Geometry check sheet. Reference: the model listing, model coordinates, mm. A direction names the side the tool comes from. Round coordinates to 2 decimals unless told otherwise and drop trailing zeros. Loops run counter-clockwise (first coordinate to the right, second up) from the corner with the lowest first, then second, coordinate; pieces in that order, holes last.
Autodesk Inventor part; units mm, degrees
ref_plane "YZ Plane" through (0, 0, 0) normal (1, 0, 0) x (0, 1, 0)
ref_plane "XZ Plane" through (0, 0, 0) normal (0, 1, 0) x (-1, 0, 0)
ref_plane "XY Plane" through (0, 0, 0) normal (0, 0, 1) x (1, 0, 0)
sketch "Sketch1" plane through (0, 0, 0) normal (0, 1, 0) x (-1, 0, 0)
  line L0 (0, 0) -> (200, 0)
  line L1 (200, 0) -> (200, 172)
  line L2 (200, 172) -> (0, 172)
  line L3 (0, 172) -> (0, 0)
  line L4 (0, 172) -> (200, 172)
  line L5 (200, 172) -> (200, -28)
  line L6 (200, -28) -> (0, -28)
  line L7 (0, -28) -> (0, 172)
  line L8 (200, 172) -> (195, 172)
  line L9 (195, 172) -> (195, 167)
  line L10 (195, 167) -> (200, 167)
  line L11 (195, 172) -> (195, 144)
  line L12 (195, 167) -> (130, 167)
  line L13 (130, 167) -> (130, 144)
  line L14 (130, 144) -> (195, 144)
  line L15 (195, 144) -> (195, 0)
  line L16 (195, 0) -> (195, 5)
  line L17 (195, 5) -> (130, 5)
  line L18 (130, 5) -> (130, 33)
  line L19 (130, 33) -> (195, 33)
  line L20 (0, 167) -> (5, 167)
  line L21 (5, 167) -> (5, 139)
  line L22 (130, 167) -> (130, 139)
  line L23 (130, 139) -> (195, 139)
  line L24 (5, 139) -> (70, 139)
  line L25 (70, 139) -> (70, 167)
  line L26 (70, 167) -> (5, 167)
  line L27 (5, 139) -> (5, 0)
  line L28 (5, 33) -> (70, 33)
  line L29 (70, 33) -> (70, 5)
  line L30 (70, 5) -> (5, 5)
  line L31 (130, 139) -> (70, 139)
  line L32 (130, 33) -> (70, 33)
  line L33 (130, 167) -> (70, 167)
  line L34 (130, 5) -> (70, 5)
  line L35 (37.5, 33) -> (37.5, 139)
  line L36 (162.5, 33) -> (162.5, 139)
  line L37 (5, 33) -> (7, 33)
  line L38 (5, 33) -> (5, 35)
  line L39 (5, 35) -> (195, 35)
  line L40 (195, 139) -> (197, 139)
  line L41 (5, 139) -> (5, 137)
  line L42 (5, 137) -> (195, 137)
  line L43 (100, 5) -> (90, 5)
  line L44 (90, 5) -> (110, 5)
  line L45 (110, 5) -> (110, 33)
  line L46 (90, 5) -> (90, 33)
  line L47 (90, 139) -> (90, 167)
  line L48 (110, 137) -> (110, 167)
  point P0 (110, 139)
  dimension "d0" = 200
  dimension "d1" = 172
  dimension "d2" = 200
  dimension "d3" = 200
  dimension "d4" = 5
  dimension "d5" = 5
  dimension "d6" = 28
  dimension "d7" = 65
  dimension "d8" = 5
  dimension "d9" = 28
  dimension "d10" = 5
  dimension "d11" = 28
  dimension "d12" = 28
  dimension "d13" = 65
  dimension "d14" = 2
  dimension "d15" = 2
  dimension "d16" = 2
  dimension "d17" = 2
  dimension "d18" = 10
  dimension "d19" = 20
extrude "Extrusion1" add sketch "Sketch1" along normal blind 145 contours L3 L20 L21 L27 L0 | L27 L30 L34 L17 L15 L0 | L3 L2 L9 L12 L33 L26 L20 | L15 L11 L10 L1 L0 | L27 L39 L35 L28 | L2 L1 L10 L9 | L24 L35 L42 L27 | L19 L36 L39 L15 | L28 L35 L39 L36 L19 L32 | L46 L32 L45 L34 | L24 L31 L48 L42 L35 | L33 L48 L31 L47 | L42 L36 L23 L15 | L48 L31 L23 L36 L42
sketch "Sketch2" plane through (0, 0, 0) normal (0, -1, 0) x (1, 0, 0)
  line L0 (-5, 137) -> (-195, 137)
  line L1 (-195, 35) -> (-5, 35)
  line L2 (-195, 137) -> (-5, 137)
  line L3 (-5, 137) -> (-5, 35)
  line L4 (-5, 35) -> (-195, 35)
  line L5 (-195, 35) -> (-195, 137)
  point P0 (0, 0)
extrude "Extrusion2" add sketch "Sketch2" against normal blind 5
sketch "Sketch3" plane through (-195, 0, 139) normal (0, 0, 1) x (1, 0, 0)
  point P0 (195, 0)
sketch "Sketch4" plane through (0, 5, 0) normal (0, 1, 0) x (1, 0, 0)
  line L0 (-90, -33) -> (-90, -5)
  line L1 (-5, -33) -> (-90, -33)
  line L2 (-90, -33) -> (-5, -33)
  line L3 (-5, -33) -> (-47.5, -33)
  line L4 (-47.5, -33) -> (-47.5, -172)
  line L5 (-200, -172) -> (0, -172)
  line L6 (-109.747, -33) -> (-194.7552, -33)
  line L7 (-194.7552, -33) -> (-109.747, -33)
  line L8 (-110, -5) -> (-110, -33)
  line L9 (-195, -5) -> (-110, -5)
  line L10 (-110, -5) -> (-195, -5)
  line L11 (-195, -5) -> (-152.5, -5)
  line L12 (-152.5, -5) -> (-152.5, -172)
  line L13 (-110, -167) -> (-195, -167)
  point P0 (0, 0)
sketch "Sketch5" plane through (-200, 0, 172) normal (0, 0, 1) x (1, 0, 0)
  line L0 (5, 144.4425) -> (89.9982, 145)
  line L1 (0, 145) -> (200, 145)
  line L2 (5, 144.4425) -> (47.1963, 145)
  line L3 (47.4991, 144.7212) -> (47.4991, 0)
  line L4 (0, 0) -> (200, 0)
  line L5 (200, 145) -> (195, 145)
  line L6 (195, 145) -> (110, 145)
  line L7 (110, 145) -> (152.5, 145)
  line L8 (152.5, 145) -> (152.5, 0)
  line L9 (195, 5) -> (5, 5)
  line L10 (152.5, 5) -> (152.5, 42.5)
  line L11 (152.5, 42.5) -> (47.4991, 42.5)
  circle A0 centre (47.4991, 42.5) radius 5
  circle A1 centre (152.5, 42.5) radius 5
  line L12 (47.4991, 47.5) -> (51.4082, 45.6174)
  line L13 (51.4082, 45.6174) -> (52.3737, 41.3874)
  line L14 (52.3737, 41.3874) -> (49.6685, 37.9952)
  line L15 (49.6685, 37.9952) -> (45.3297, 37.9952)
  line L16 (45.3297, 37.9952) -> (42.6244, 41.3874)
  line L17 (42.6244, 41.3874) -> (43.5899, 45.6174)
  line L18 (43.5899, 45.6174) -> (47.4991, 47.5)
  line L19 (152.5, 47.5) -> (156.4092, 45.6174)
  line L20 (156.4092, 45.6174) -> (157.3746, 41.3874)
  line L21 (157.3746, 41.3874) -> (154.6694, 37.9952)
  line L22 (154.6694, 37.9952) -> (150.3306, 37.9952)
  line L23 (150.3306, 37.9952) -> (147.6254, 41.3874)
  line L24 (147.6254, 41.3874) -> (148.5908, 45.6174)
  line L25 (148.5908, 45.6174) -> (152.5, 47.5)
  dimension "d29" = 10
  dimension "d30" = 10
  dimension "d24" = 85
  dimension "d25" = 42.2
  dimension "d26" = 5
  dimension "d27" = 85
  dimension "d28" = 37.5
extrude "Extrusion3" cut sketch "Sketch5" against normal blind 376.75 contours L12 L13 L11 L3 | L3 L15 L16 L17 L18 | L11 L13 L14 L15 L3 | L19 L20 L21 L22 L8 | L8 L11 L24 L25 | L8 L22 L23 L24 L11
sketch "Sketch6" plane through (0, 145, 0) normal (0, 1, 0) x (1, 0, 0)
  line L0 (-110, -5) -> (-110, -33)
  line L1 (-110, -5) -> (-110, -162.1983)
  line L2 (-110, -162.1983) -> (-90, -162.1983)
  line L3 (-90, -167) -> (-90, -139)
  line L4 (-90, -162.1983) -> (-90, -32.5425)
  line L5 (-90, -32.5425) -> (-110, -32.5425)
  line L6 (-195, -35) -> (-5, -35)
  line L7 (-110, -35) -> (-110, -50)
  line L8 (-110, -50) -> (-90, -50)
  line L9 (-90, -50) -> (-90, -35)
  line L10 (-5, -137) -> (-195, -137)
  line L11 (-90, -137) -> (-90, -122)
  line L12 (-90, -122) -> (-110, -122)
  point P0 (0, 0)
  point P1 (-110, -137)
  dimension "d33" = 15
  dimension "d34" = 15
extrude "Extrusion4" add sketch "Sketch6" against normal blind 144.75 contours L6 L4 L8 L1 | L12 L4 L10 L1
1) Access from +Z, -Z, +X, -X, +Y, -Y to the whole of each face (thin tool, end or side, straight path). Record for faces 1 (the face through (-47, 71, 33)), 2 (the face through (-90, 76, 43)), 3 (the face through (-101, 0, 87)).
Report:
face 1: +Y, -Y
face 2: +Y
face 3: +Z, -Z, +X, -X, -Y
2) Sectioned sample at A-A, the plane x = -144.5. Record the cut outline in (y, z), then the cut area to 3 significant figures.
Report:
outline: (0, 0) - (145, 0) - (145, 5) - (0, 5) - close; (0, 33) - (145, 33) - (145, 35) - (5, 35) - (5, 137) - (145, 137) - (145, 139) - (0, 139) - close; (0, 167) - (145, 167) - (145, 172) - (0, 172) - close
area: 2,540 mm2
3) Gauge pin test, flat ends, axial feed: pin 1 (12 mm diameter, centred on y = 117.5, z = 45, fed in from +X); pin 2 (3 mm diameter, centred on x = -78.5, z = 84.5, fed in from +Y). Record the tip position at first contact, or that the pin passes through.
Report:
pin 1: stops at x = 0
pin 2: stops at y = 5
4) Sectioned sample at B-B, the plane y = 56.5. State how many separate pieces and enclosed holes the cut face has, then the cut area to 3 significant figures.
Report:
separate pieces: 1
enclosed holes: 5
area: 6,100 mm2
5) Sectioned sample at C-C, the plane z = 103. Record the cut outline in (x, y), then the cut area to 3 significant figures.
Report:
outline: (-200, 0) - (0, 0) - (0, 145) - (-5, 145) - (-5, 5) - (-195, 5) - (-195, 145) - (-200, 145) - close
area: 2,400 mm2
6) Sectioned sample at D-D, the plane x = -106. Record the cut outline in (y, z).
Report:
outline: (0, 0) - (145, 0) - (145, 50) - (5, 50) - (5, 122) - (145, 122) - (145, 172) - (0, 172) - close
7) Mould release check, pull along X, two halves, no side actions. Record for faces 4 (the face through (-200, 71, 85)), 5 (the face through (-100, 145, 125)), 6 (the face through (-5, 71, 153)): +X half, -X half, draft (parallel to the pull), parting line (faces both ways), or undercut.
Report:
face 4: -X half
face 5: draft
face 6: undercut
8) Scan lines: line 1 along X through (y, z) = (131, 18.5); line 2 along Z through (x, y) = (-82, 105.5); line 3 along X through (y, z) = (88, 52). Record each from-to range of solid material in increasing order.
Report:
line 1: x = -200 to -195, -110 to -90, -5 to 0
line 2: z = 0 to 5, 33 to 35, 137 to 139, 167 to 172
line 3: x = -200 to -195, -5 to 0
